Read the model definition and answer for the solid it produces. Units are mm, in the model's axes. Coordinates: 2 decimals unless noted, no trailing zeros. Order: outer loops, then holes, each group sorted by start corner. A loop starts at its lowest first (then second) coordinate and runs counter-clockwise, first axis right, second up. Notation, with made-up numbers: M 58.25,78 L 84.25,78 A19 ccw 84.25,94 Z; hole C 78,61.25 d2. An arc over 180 degrees is marked long. Use a Markdown table: item, result. Add a question column.
1) Find section A-A on x = 0.15. Write down the section's boundary in (y, z).
2) This flat-tipped pin is pushed along its axis until it touches: pin 1 Ø1.5 at (y, z) = (9.5, 1) entering from -X. Where does it stop, or does it pass through?
3) Find the intervals of material crossed by probe 1 along Z at (x, y) = (0.6, 2.5); probe 2 along Z at (x, y) = (0.6, 5.75); probe 3 along Y at (x, z) = (0.7, 1), in increasing order. Write a range as [from, to].
Autodesk Inventor part; units mm, degrees
ref_plane "YZ Plane" through (0, 0, 0) normal (1, 0, 0) x (0, 1, 0)
ref_plane "XZ Plane" through (0, 0, 0) normal (0, 1, 0) x (-1, 0, 0)
ref_plane "XY Plane" through (0, 0, 0) normal (0, 0, 1) x (1, 0, 0)
sketch "Sketch1" plane through (0, 0, 0) normal (1, 0, 0) x (0, 1, 0)
  spline S0 degree 3 poles (-4.479, -27.0431) (-4.7662, -26.7746) (-5.439, -26.5061) (-6.0629, -26.2376) (-6.6869, -25.9691) (-7.2127, -25.7006) (-7.3009, -25.4322) (-7.389, -25.1637) (-7.0326, -24.8952) (-6.4617, -24.6267) (-5.8908, -24.3582) (-5.1506, -24.0897) (-4.7189, -23.8212) (-4.2873, -23.5527) (-4.1983, -23.2842) (-4.5096, -23.0157) (-4.8208, -22.7472) (-5.5075, -22.4787) (-6.1264, -22.2102) (-6.7453, -21.9417) (-7.2474, -21.6732) (-7.3085, -21.4047) (-7.3696, -21.1362) (-6.9849, -20.8677) (-6.4028, -20.5992) (-5.8207, -20.3307) (-5.0872, -20.0622) (-4.6758, -19.7937) (-4.2645, -19.5252) (-4.2079, -19.2568) (-4.5426, -18.9883) (-4.8772, -18.7198) (-5.5767, -18.4513) (-6.1893, -18.1828) (-6.802, -17.9143) (-7.2794, -17.6458) (-7.3133, -17.3773) (-7.3473, -17.1088) (-6.935, -16.8403) (-6.3428, -16.5718) (-5.7505, -16.3033) (-5.0251, -16.0348) (-4.6349, -15.7663) (-4.2446, -15.4978) (-4.2205, -15.2293) (-4.5779, -14.9608) (-4.9354, -14.6923) (-5.6463, -14.4238) (-6.2516, -14.1553) (-6.8569, -13.8868) (-7.3087, -13.6183) (-7.3154, -13.3498) (-7.3221, -13.0814) (-6.8831, -12.8129) (-6.2818, -12.5444) (-5.6805, -12.2759) (-4.9645, -12.0074) (-4.5961, -11.7389) (-4.2277, -11.4704) (-4.236, -11.2019) (-4.6156, -10.9334) (-4.9952, -10.6649) (-5.7162, -10.3964) (-6.313, -10.1279) (-6.9098, -9.8594) (-7.3353, -9.5909) (-7.3147, -9.3224) (-7.2941, -9.0539) (-6.8291, -8.7854) (-6.22, -8.5169) (-5.6108, -8.2484) (-4.9055, -7.9799) (-4.5596, -7.7114) (-4.2137, -7.4429) (-4.2544, -7.1745) (-4.6555, -6.906) (-5.0566, -6.6375) (-5.7863, -6.369) (-6.3735, -6.1005) (-6.9607, -5.832) (-7.359, -5.5635) (-7.3112, -5.295) (-7.2634, -5.0265) (-6.7733, -4.758) (-6.1573, -4.4895) (-5.5414, -4.221) (-4.8482, -3.9525) (-4.5255, -3.684) (-4.2027, -3.4155) (-4.2758, -3.147) (-4.6975, -2.8785) (-5.1193, -2.61) (-5.8564, -2.3415) (-6.433, -2.073) (-7.0095, -1.8045) (-7.3799, -1.536) (-7.3049, -1.2675) (-7.23, -0.9991) (-6.7157, -0.7306) (-6.0941, -0.4621) (-5.4725, -0.1936) (-4.7927, 0.0749) (-4.4937, 0.3434) (-4.1946, 0.6119) (-4.3, 0.8804) (-4.7417, 1.1489) (-5.1834, 1.4174) (-5.9265, 1.6859) (-6.4913, 1.9544) (-7.0561, 2.2229) (-7.3978, 2.4914) (-7.2959, 2.7599) (-7.194, 3.0284) (-6.6565, 3.2969) (-6.0304, 3.5654) (-5.4043, 3.8339) (-4.7391, 4.1024) (-4.4644, 4.3709) (-4.1896, 4.6394) (-4.327, 4.9079) (-4.7878, 5.1763) (-5.2486, 5.4448) (-5.9964, 5.7133) (-6.5483, 5.9818) (-7.1003, 6.2503) (-7.4128, 6.5188) (-7.2841, 6.7873) (-7.1554, 7.0558) (-6.5956, 7.3243) (-5.9662, 7.5928) (-5.3368, 7.8613) (-4.6875, 8.1298) (-4.4375, 8.3983) (-4.1876, 8.6668) (-4.3567, 8.9353) (-4.8358, 9.2038) (-5.3148, 9.4723) (-6.0659, 9.7408) (-6.604, 10.0093) (-7.1422, 10.2778) (-7.4249, 10.5463) (-7.2696, 10.8148) (-7.1143, 11.0832) (-6.5334, 11.3517) (-5.9018, 11.6202) (-5.2702, 11.8887) (-4.638, 12.1572) (-4.4133, 12.4257) (-4.1886, 12.6942) (-4.3892, 12.9627) (-4.8856, 13.2312) (-5.382, 13.4997) (-6.135, 13.7682) (-6.6583, 14.0367) (-7.1816, 14.3052) (-7.434, 14.5737) (-7.2524, 14.8422) (-7.0708, 15.1107) (-6.4697, 15.3792) (-5.8372, 15.6477) (-5.2046, 15.9162) (-4.5906, 16.1847) (-4.3916, 16.4532) (-4.1926, 16.7217) (-4.4244, 16.9902) (-4.9372, 17.2586) (-5.45, 17.5271) (-6.2034, 17.7956) (-6.711, 18.0641) (-7.2185, 18.3326) (-7.44, 18.6011) (-7.2325, 18.8696) (-7.025, 19.1381) (-6.4049, 19.4066) (-5.7725, 19.6751) (-5.1402, 19.9436) (-4.5456, 20.2121) (-4.3726, 20.4806) (-4.1997, 20.7491) (-4.4621, 21.0176) (-4.9904, 21.2861) (-5.5187, 21.5546) (-6.2712, 21.8231) (-6.762, 22.0916) (-7.2528, 22.3601) (-7.4431, 22.6286) (-7.21, 22.8971) (-6.977, 23.1656) (-6.339, 23.434) (-5.708, 23.7025) (-5.077, 23.971) (-4.5029, 24.2395) (-4.3563, 24.508) (-4.3292, 24.5576) (-4.3155, 24.6073) (-4.3155, 24.6569) knots -81.21017 -81.21017 -81.21017 -81.21017 -79.944914 -79.944914 -79.944914 -78.679659 -78.679659 -78.679659 -77.414403 -77.414403 -77.414403 -76.149147 -76.149147 -76.149147 -74.883892 -74.883892 -74.883892 -73.618636 -73.618636 -73.618636 -72.35338 -72.35338 -72.35338 -71.088125 -71.088125 -71.088125 -69.822869 -69.822869 -69.822869 -68.557613 -68.557613 -68.557613 -67.292358 -67.292358 -67.292358 -66.027102 -66.027102 -66.027102 -64.761846 -64.761846 -64.761846 -63.496591 -63.496591 -63.496591 -62.231335 -62.231335 -62.231335 -60.96608 -60.96608 -60.96608 -59.700824 -59.700824 -59.700824 -58.435568 -58.435568 -58.435568 -57.170313 -57.170313 -57.170313 -55.905057 -55.905057 -55.905057 -54.639801 -54.639801 -54.639801 -53.374546 -53.374546 -53.374546 -52.10929 -52.10929 -52.10929 -50.844034 -50.844034 -50.844034 -49.578779 -49.578779 -49.578779 -48.313523 -48.313523 -48.313523 -47.048267 -47.048267 -47.048267 -45.783012 -45.783012 -45.783012 -44.517756 -44.517756 -44.517756 -43.2525 -43.2525 -43.2525 -41.987245 -41.987245 -41.987245 -40.721989 -40.721989 -40.721989 -39.456733 -39.456733 -39.456733 -38.191478 -38.191478 -38.191478 -36.926222 -36.926222 -36.926222 -35.660966 -35.660966 -35.660966 -34.395711 -34.395711 -34.395711 -33.130455 -33.130455 -33.130455 -31.865199 -31.865199 -31.865199 -30.599944 -30.599944 -30.599944 -29.334688 -29.334688 -29.334688 -28.069432 -28.069432 -28.069432 -26.804177 -26.804177 -26.804177 -25.538921 -25.538921 -25.538921 -24.273665 -24.273665 -24.273665 -23.00841 -23.00841 -23.00841 -21.743154 -21.743154 -21.743154 -20.477898 -20.477898 -20.477898 -19.212643 -19.212643 -19.212643 -17.947387 -17.947387 -17.947387 -16.682131 -16.682131 -16.682131 -15.416876 -15.416876 -15.416876 -14.15162 -14.15162 -14.15162 -12.886364 -12.886364 -12.886364 -11.621109 -11.621109 -11.621109 -10.355853 -10.355853 -10.355853 -9.090597 -9.090597 -9.090597 -7.825342 -7.825342 -7.825342 -6.560086 -6.560086 -6.560086 -5.29483 -5.29483 -5.29483 -4.029575 -4.029575 -4.029575 -2.764319 -2.764319 -2.764319 -1.499063 -1.499063 -1.499063 -0.233808 -0.233808 -0.233808 0 0 0 0
  spline S1 degree 3 poles (-4.3155, 25.6569) (-4.3155, 25.3884) (-4.761, 25.1199) (-5.3643, 24.8514) (-5.9676, 24.5829) (-6.6811, 24.3144) (-7.044, 24.0459) (-7.407, 23.7774) (-7.3908, 23.5089) (-7.0058, 23.2404) (-6.6209, 22.9719) (-5.8977, 22.7034) (-5.3031, 22.4349) (-4.7085, 22.1664) (-4.2896, 21.8979) (-4.3169, 21.6294) (-4.3441, 21.3609) (-4.8154, 21.0925) (-5.4263, 20.824) (-6.0373, 20.5555) (-6.7397, 20.287) (-7.08, 20.0185) (-7.4203, 19.75) (-7.3716, 19.4815) (-6.9654, 19.213) (-6.5592, 18.9445) (-5.8275, 18.676) (-5.2428, 18.4075) (-4.6581, 18.139) (-4.2666, 17.8705) (-4.3211, 17.602) (-4.3755, 17.3335) (-4.8716, 17.065) (-5.4891, 16.7965) (-6.1066, 16.528) (-6.7965, 16.2595) (-7.1136, 15.991) (-7.4306, 15.7225) (-7.3496, 15.454) (-6.9228, 15.1855) (-6.4961, 14.9171) (-5.7574, 14.6486) (-5.1836, 14.3801) (-4.6099, 14.1116) (-4.2465, 13.8431) (-4.328, 13.5746) (-4.4096, 13.3061) (-4.9297, 13.0376) (-5.5525, 12.7691) (-6.1753, 12.5006) (-6.8516, 12.2321) (-7.1447, 11.9636) (-7.4379, 11.6951) (-7.3247, 11.4266) (-6.8782, 11.1581) (-6.4318, 10.8896) (-5.6874, 10.6211) (-5.1256, 10.3526) (-4.5639, 10.0841) (-4.2292, 9.8156) (-4.3377, 9.5471) (-4.4462, 9.2786) (-4.9893, 9.0101) (-5.6163, 8.7417) (-6.2434, 8.4732) (-6.9047, 8.2047) (-7.1735, 7.9362) (-7.4422, 7.6677) (-7.297, 7.3992) (-6.8316, 7.1307) (-6.3663, 6.8622) (-5.6176, 6.5937) (-5.0689, 6.3252) (-4.5202, 6.0567) (-4.2149, 5.7882) (-4.3502, 5.5197) (-4.4854, 5.2512) (-5.0505, 4.9827) (-5.6806, 4.7142) (-6.3106, 4.4457) (-6.9558, 4.1772) (-7.1996, 3.9087) (-7.4434, 3.6402) (-7.2665, 3.3717) (-6.7832, 3.1032) (-6.2998, 2.8348) (-5.5481, 2.5663) (-5.0135, 2.2978) (-4.4789, 2.0293) (-4.2036, 1.7608) (-4.3654, 1.4923) (-4.5271, 1.2238) (-5.1131, 0.9553) (-5.7451, 0.6868) (-6.377, 0.4183) (-7.0048, 0.1498) (-7.2233, -0.1187) (-7.4417, -0.3872) (-7.2334, -0.6557) (-6.7329, -0.9242) (-6.2324, -1.1927) (-5.4792, -1.4612) (-4.9597, -1.7297) (-4.4401, -1.9982) (-4.1953, -2.2667) (-4.3832, -2.5352) (-4.5712, -2.8037) (-5.177, -3.0722) (-5.8097, -3.3406) (-6.4423, -3.6091) (-7.0516, -3.8776) (-7.2443, -4.1461) (-7.4369, -4.4146) (-7.1976, -4.6831) (-6.6809, -4.9516) (-6.1642, -5.2201) (-5.4109, -5.4886) (-4.9074, -5.7571) (-4.4039, -6.0256) (-4.19, -6.2941) (-4.4038, -6.5626) (-4.6176, -6.8311) (-5.2422, -7.0996) (-5.8743, -7.3681) (-6.5064, -7.6366) (-7.0961, -7.9051) (-7.2626, -8.1736) (-7.4291, -8.4421) (-7.1593, -8.7106) (-6.6273, -8.9791) (-6.0954, -9.2476) (-5.3433, -9.516) (-4.8568, -9.7845) (-4.3702, -10.053) (-4.1877, -10.3215) (-4.4269, -10.59) (-4.6662, -10.8585) (-5.3083, -11.127) (-5.9388, -11.3955) (-6.5693, -11.664) (-7.1382, -11.9325) (-7.2783, -12.201) (-7.4183, -12.4695) (-7.1185, -12.738) (-6.5722, -13.0065) (-6.026, -13.275) (-5.2767, -13.5435) (-4.808, -13.812) (-4.3393, -14.0805) (-4.1884, -14.349) (-4.4526, -14.6175) (-4.7169, -14.886) (-5.3754, -15.1545) (-6.0031, -15.4229) (-6.6308, -15.6914) (-7.1779, -15.9599) (-7.2912, -16.2284) (-7.4046, -16.4969) (-7.0752, -16.7654) (-6.5157, -17.0339) (-5.9563, -17.3024) (-5.211, -17.5709) (-4.761, -17.8394) (-4.3111, -18.1079) (-4.1921, -18.3764) (-4.4809, -18.6449) (-4.7697, -18.9134) (-5.4434, -19.1819) (-6.067, -19.4504) (-6.6907, -19.7189) (-7.215, -19.9874) (-7.3014, -20.2559) (-7.3879, -20.5244) (-7.0296, -20.7929) (-6.4579, -21.0614) (-5.8863, -21.3299) (-5.1464, -21.5983) (-4.7161, -21.8668) (-4.2857, -22.1353) (-4.1989, -22.4038) (-4.5116, -22.6723) (-4.8244, -22.9408) (-5.512, -23.2093) (-6.1305, -23.4778) (-6.749, -23.7463) (-7.2495, -24.0148) (-7.3089, -24.2833) (-7.3682, -24.5518) (-6.9818, -24.8203) (-6.3989, -25.0888) (-5.8161, -25.3573) (-5.0831, -25.6258) (-4.6731, -25.8943) (-4.2631, -26.1628) (-4.2086, -26.4313) (-4.5448, -26.6998) (-4.6881, -26.8142) (-4.8942, -26.9287) (-5.1345, -27.0431) knots 0 0 0 0 1.265256 1.265256 1.265256 2.530511 2.530511 2.530511 3.795767 3.795767 3.795767 5.061023 5.061023 5.061023 6.326278 6.326278 6.326278 7.591534 7.591534 7.591534 8.85679 8.85679 8.85679 10.122045 10.122045 10.122045 11.387301 11.387301 11.387301 12.652557 12.652557 12.652557 13.917812 13.917812 13.917812 15.183068 15.183068 15.183068 16.448324 16.448324 16.448324 17.713579 17.713579 17.713579 18.978835 18.978835 18.978835 20.244091 20.244091 20.244091 21.509346 21.509346 21.509346 22.774602 22.774602 22.774602 24.039858 24.039858 24.039858 25.305113 25.305113 25.305113 26.570369 26.570369 26.570369 27.835625 27.835625 27.835625 29.10088 29.10088 29.10088 30.366136 30.366136 30.366136 31.631392 31.631392 31.631392 32.896647 32.896647 32.896647 34.161903 34.161903 34.161903 35.427159 35.427159 35.427159 36.692414 36.692414 36.692414 37.95767 37.95767 37.95767 39.222926 39.222926 39.222926 40.488181 40.488181 40.488181 41.753437 41.753437 41.753437 43.018693 43.018693 43.018693 44.283948 44.283948 44.283948 45.549204 45.549204 45.549204 46.814459 46.814459 46.814459 48.079715 48.079715 48.079715 49.344971 49.344971 49.344971 50.610226 50.610226 50.610226 51.875482 51.875482 51.875482 53.140738 53.140738 53.140738 54.405993 54.405993 54.405993 55.671249 55.671249 55.671249 56.936505 56.936505 56.936505 58.20176 58.20176 58.20176 59.467016 59.467016 59.467016 60.732272 60.732272 60.732272 61.997527 61.997527 61.997527 63.262783 63.262783 63.262783 64.528039 64.528039 64.528039 65.793294 65.793294 65.793294 67.05855 67.05855 67.05855 68.323806 68.323806 68.323806 69.589061 69.589061 69.589061 70.854317 70.854317 70.854317 72.119573 72.119573 72.119573 73.384828 73.384828 73.384828 74.650084 74.650084 74.650084 75.91534 75.91534 75.91534 77.180595 77.180595 77.180595 78.445851 78.445851 78.445851 79.711107 79.711107 79.711107 80.976362 80.976362 80.976362 82.241618 82.241618 82.241618 82.780966 82.780966 82.780966 82.780966
  line L0 (-4.7597, 6.1899) -> (4.004, 2.288)
  line L1 (-5.1314, 6.3554) -> (4.8686, 6.3554) construction
  line L2 (-5.1314, 5.355) -> (3.6323, 1.4531)
  line L3 (-5.1314, 5.355) -> (4.8686, 5.355) construction
  line L4 (4.004, 2.288) -> (3.6323, 1.4531)
  line L5 (-5.1314, 5.355) -> (-4.7597, 6.1899)
  point P0 (0, 0)
  dimension "d1" = 24
  dimension "d3" = 24
extrude "Extrusion1" add sketch "Sketch1" along normal blind 0.914 contours L5 S1 L2 | S1 L5 L0 L4 L2
sketch "Sketch2" plane through (0, 4.004, 2.288) normal (0, 0.9135455, -0.4067366) x (1, 0, 0)
  line L0 (0, 0.9139) -> (0, 0)
  line L1 (0, 0) -> (0.914, 0)
  line L2 (0.914, 0.9139) -> (0.914, 0)
  line L3 (0, 0.9139) -> (0.914, 0.9139)
  line L4 (0.457, 0.9139) -> (0.457, 0) construction
  line L5 (0.914, 0.457) -> (0, 0.457) construction
  circle A0 centre (0.457, 0.457) radius 0.457
extrude "Extrusion2" cut sketch "Sketch2" against normal blind 20 contours L3 A0 L0 | A0 L1 L0 | L3 L2 A0 | A0 L2 L1
sketch "Sketch3" plane through (0.457, 3.8182, 1.8706) normal (0, 0.9135455, -0.4067366) x (1, 0, 0)
  circle A0 centre (0, 0) radius 0.457
  circle A1 centre (0, 0) radius 0.457
  point P0 (-0.457, 3.2618)
extrude "Extrusion3" add sketch "Sketch3" along normal blind 8.75
properties part number "Carriage Tooth"
Check result:
| question | item | result |
|---|---|---|
| 1 | outline | M -5.08,5.46 L 11.67,-2 L 11.95,-1.38 L -4.81,6.08 Z |
| 2 | pin 1 | passes through |
| 3 | probe 1 | z = [1.98, 2.93] |
| 3 | probe 2 | z = [0.54, 1.49] |
| 3 | probe 3 | y = [4.82, 6.73] |
